```python
from build123d import *

# Parameters (mm, degrees)
SKETCH1_W           = 15
SKETCH1_H           = 15
BOSS_EXTRUDE1_DEPTH = 30
BOSS_EXTRUDE2_DEPTH = 15
BOSS_EXTRUDE3_DEPTH = 15
FILLET1_R           = 5
FILLET2_R           = 5
FILLET3_R           = 5
FILLET4_R           = 5
FILLET5_R           = 10


with BuildPart() as part:
    # Sketch1 → Boss-Extrude1 (new body)
    with BuildSketch(Plane.XY):
        Rectangle(SKETCH1_W, SKETCH1_H)
    extrude(amount=BOSS_EXTRUDE1_DEPTH)

    # Sketch2 → Boss-Extrude2 (add)
    with BuildSketch(Plane(origin=(7.5, 0, 0), x_dir=(0, 0, -1), z_dir=(1, 0, 0))):
        Polygon((0, 7.5), (0, -7.5), (15, 7.5), (21.545785732, 27.742247112), (26.510349476, 27.742247112), (26.510349476, 32.414777695), (26.510349476, 41.912857566), (18.236076569, 32.414777695), (15, 21.844799658), (8.988359791, 21.844799658), align=None)
    extrude(amount=-BOSS_EXTRUDE2_DEPTH)

    # Sketch3 → Boss-Extrude3 (add)
    with BuildSketch(Plane(origin=(0, 0, -26.510349476), x_dir=(-1, 0, 0), z_dir=(0, 0, -1))):
        Polygon((-7.5, 27.742247112), (-22.495127837, 34.382116855), (-35.622841112, 44.261996271), (-35.622841112, 55.90842978), (-22.495127837, 55.685698079), (7.5, 41.912857566), (7.5, 27.742247112), align=None)
    extrude(amount=BOSS_EXTRUDE3_DEPTH)

    # Fillet1
    fillet1_edges = [part.edges().sort_by_distance(p)[0] for p in [
        (35.622841112, 55.90842978, -34.010349476),
    ]]
    fillet(fillet1_edges, radius=FILLET1_R)

    # Fillet2
    # the kernel refuses this fillet: 5 mm, written as the material it takes off along each edge
    with BuildSketch(Plane(origin=(-7.467478677, 11.832344997, -41.510349476), x_dir=(0, 0, 1), z_dir=(0.7990028403879673, 0.6013272495504927, 0))) as fillet2_piece_1:
        with BuildLine():
            CenterArc((FILLET2_R, -FILLET2_R), FILLET2_R, 90, 90)
            Line((0, -FILLET2_R), (0, 0))
            Line((0, 0), (FILLET2_R, 0))
        make_face()
    extrude(amount=66.430120909, mode=Mode.SUBTRACT)
    with BuildSketch(Plane(origin=(22.495127837, 34.382116855, -25.077185007), x_dir=(0.7990028403879682, 0.6013272495504913, 0), z_dir=(0, 0, -1))) as fillet2_piece_2:
        with BuildLine():
            CenterArc((FILLET2_R * 0.11465315755, -FILLET2_R), FILLET2_R, 90, 13.081164811)
            Line((-FILLET2_R * 0.111677956622, -FILLET2_R * 0.0259495768916), (0, 0))
            Line((0, 0), (FILLET2_R * 0.11465315755, 0))
        make_face()
    extrude(amount=17.866328939, mode=Mode.SUBTRACT)
    with BuildSketch(Plane(origin=(-7.467478677, 11.832344997, -26.510349476), x_dir=(-0.6013272495504927, 0.7990028403879673, 0), z_dir=(0.7990028403879673, 0.6013272495504927, 0))) as fillet2_piece_3_section:
        with BuildLine():
            CenterArc((FILLET2_R, -FILLET2_R), FILLET2_R, 90, 90)
            Line((0, -FILLET2_R), (0, 0))
            Line((0, 0), (FILLET2_R, 0))
        make_face()
    fillet2_piece_3 = extrude(amount=66.430120909, mode=Mode.PRIVATE)
    fillet2_piece_3 = split(fillet2_piece_3, bisect_by=Plane(origin=(7.5, 11.832344997, -26.510349476), z_dir=(1, 0, 0)), keep=Keep.TOP, mode=Mode.PRIVATE)
    add(fillet2_piece_3, mode=Mode.SUBTRACT)
    with BuildSketch(Plane(origin=(35.622841112, 44.261996271, -20.2733136), x_dir=(0, 1, 0), z_dir=(0, 0, -1))) as fillet2_piece_4:
        with BuildLine():
            CenterArc((FILLET2_R * 0.498962870089, -FILLET2_R), FILLET2_R, 90, 53.03498585)
            Line((-FILLET2_R * 0.300039970299, -FILLET2_R * 0.39867275045), (0, 0))
            Line((0, 0), (FILLET2_R * 0.498962870089, 0))
        make_face()
    extrude(amount=27.474071752, mode=Mode.SUBTRACT)

    # Fillet3
    fillet3_edges = [part.edges().sort_by_distance(p)[0] for p in [
        (0, 7.5, -15),
        (7.5, 0, -7.5),
        (-7.5, 0, -7.5),
        (0, -7.5, 0),
    ]]
    fillet(fillet3_edges, radius=FILLET3_R)

    # Fillet4
    fillet4_edges = [part.edges().sort_by_distance(p)[0] for p in [
        (0, 21.844799658, -8.988359791),
        (7.5, 14.672399829, -4.494179896),
        (-7.5, 14.672399829, -4.494179896),
        (0, 7.5, 0),
        (-7.5, 7.5, 15),
        (7.5, 7.5, 15),
    ]]
    fillet(fillet4_edges, radius=FILLET4_R)

    # Fillet5
    fillet5_edges = [part.edges().sort_by_distance(p)[0] for p in [
        (0, 32.414777695, -18.236076569),
    ]]
    fillet(fillet5_edges, radius=FILLET5_R)


solid = part.part
```
Check sheet for the modelled part. Datum: model origin and axes. Units: mm. A direction names the side the tool comes from. Round coordinates to 2 decimals unless told otherwise and drop trailing zeros. Write each loop counter-clockwise with the first axis right and the second up, starting at its lowest first coordinate (ties: lowest second). Pieces come first, ordered by that corner, then holes. Notation, with made-up numbers: (-15, 5.5) -> (39, 5.5) arc R10 cw to (39, 24.5) -> close; hole circle Ø5 at (85, 28.5). An arc over 180 degrees is marked (long way). Put each result on its own line as item: value.
(1) Sectioned sample at D-D (z = -24). Enter the section's corners in (x, y), plus the area to 3 significant figures.
Values found:
outline: (-7.5, 27.74) -> (7.5, 27.74) -> (7.5, 39.03) -> (-7.5, 39.03) -> close
area: 169 mm^2
(2) Go/stop test with flat-tipped pins: pin 1 Ø24.5 at (y, z) = (11, -8) entering from +X; pin 2 Ø1 at (x, y) = (2.5, 6.5) entering from -Z; pin 3 Ø21 at (x, y) = (10.5, 40.5) entering from +Z; pin 4 Ø10 at (x, z) = (13, -11.5) entering from -Y. Record where each tip stops, or that it passes through.
Values found:
pin 1: stops at x = 7.5
pin 2: stops at z = -14.47
pin 3: stops at z = -17.63
pin 4: passes through
(3) Sectioned sample at C-C (y = 25). Enter the section's corners in (x, z).
Values found:
outline: (-7.5, -20.66) -> (7.5, -20.66) -> (7.5, -15.97) -> (-7.5, -15.97) -> close
(4) Sectioned sample at A-A (z = 17). Enter the section's corners in (x, y), plus the area to 3 significant figures.
Values found:
outline: (-7.5, -7.5) -> (7.5, -7.5) -> (7.5, 2.5) arc R5 ccw to (2.5, 7.5) -> (-2.5, 7.5) arc R5 ccw to (-7.5, 2.5) -> close
area: 214 mm^2
(5) Material ranges on line 1 (X direction, y = 36.5, z = -25); line 2 (Z direction, x = 20, y = 51.5); line 3 (Z direction, x = -1, y = 3), recorded low to high.
Values found:
line 1: x = -7.5 to 7.5
line 2: z = -41.51 to -26.51
line 3: z = -10.5 to 30
(6) Tool access check on faces 1 (the face through (0, 7.5, 16)), 2 (the face through (0.105, 18.06, -18.415)). Record the directions out of +Z, -Z, +X, -X, +Y, -Y that give a thin tool (end or side, any length) a straight path to the whole face; none if there is none.
Values found:
face 1: +Z, +X, -X, +Y
face 2: -Z, +X, -X, -Y
(7) Sectioned sample at B-B (x = 3.5). Enter the section's corners in (y, z), plus the area to 3 significant figures.
Values found:
outline: (-7.5, 2.07) arc R5 ccw to (-6.67, -0.69) -> (7.43, -14.78) arc R5 ccw to (8.65, -15.37) -> (27.74, -21.55) -> (27.74, -41.51) -> (46.96, -41.51) -> (46.96, -26.51) -> (41.91, -26.51) -> (34.02, -19.63) arc R10 ccw to (30.38, -17.61) -> (21.84, -15) -> (21.84, -11.76) arc R5 ccw to (20.29, -8.14) -> (9.79, -1.56) arc R5.1 cw to (7.4, 2.77) -> (7.4, 30) -> (-7.5, 30) -> close
area: 1,140 mm^2
